Geometry check sheet. Reference: drawing and pictorial views, mm from the part's lowest x, y, z. Round coordinates to 2 decimals unless told otherwise and drop trailing zeros. Write each loop counter-clockwise with the first axis right and the second up, starting at its lowest first coordinate (ties: lowest second). Pieces come first, ordered by that corner, then holes. Notation, with made-up numbers: M 77,38.25 L 128,38.25 A34 cw 128,76.25 Z; hole C -5,85.5 d5. An arc over 180 degrees is marked long. Answer in a Markdown table with one row per item. Add a question column.
1. Material ranges on probe 1 along Z at (x, y) = (38.16, 2.05); probe 2 along X at (y, z) = (0.9, 69); probe 3 along X at (y, z) = (2.55, 71.5), recorded low to high.
2. Go/stop test with flat-tipped pins: pin 1 Ø4 at (x, z) = (50, 31) entering from -Y; pin 2 Ø4.5 at (x, z) = (10.949, 69.94) entering from -Y. Record where each tip stops, or that it passes through.
3. Sectioned sample at B-B on x = 38.16. Record the cut outline in (y, z), plus the area to 3 significant figures.
4. Sectioned sample at A-A on z = 69.94. Record the cut outline in (x, y), plus the area to 3 significant figures.
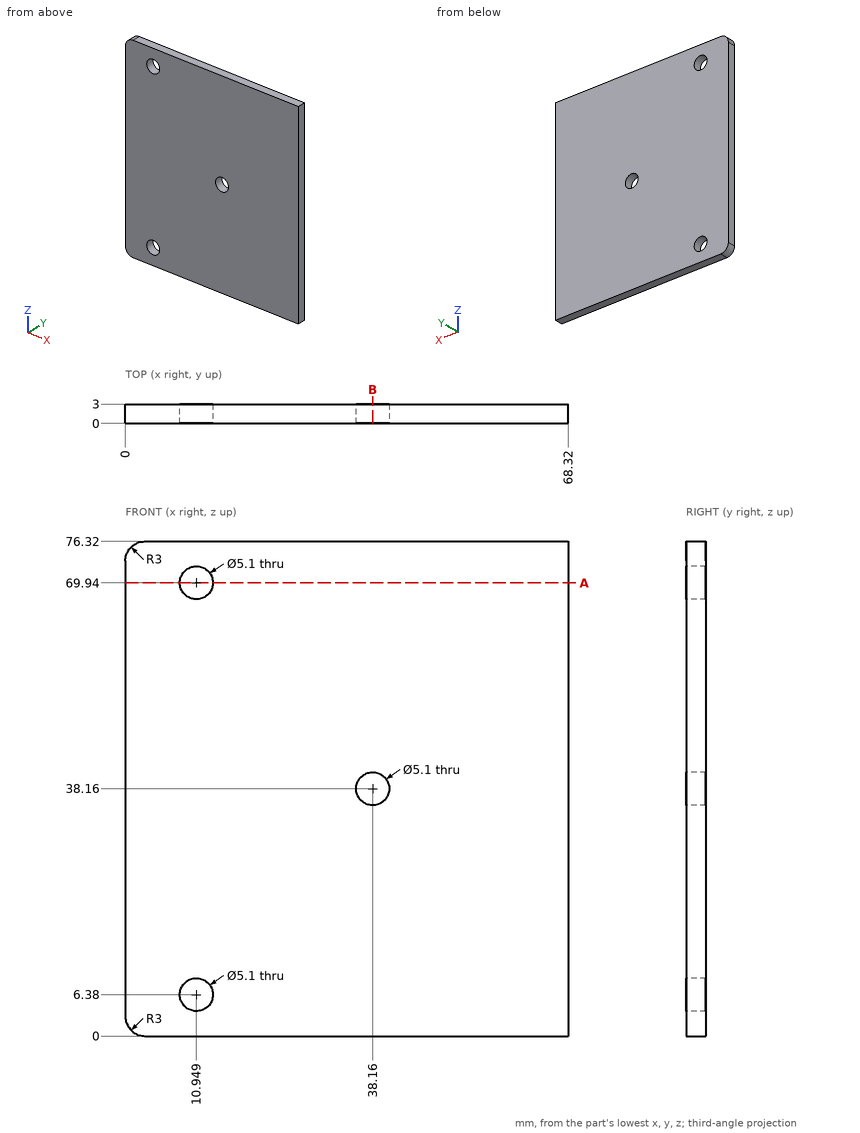
Geometry check:
| question | item | result |
|---|---|---|
| 1 | probe 1 | z = 0 to 35.61, 40.71 to 76.32 |
| 1 | probe 2 | x = 0 to 8.58, 13.32 to 68.32 |
| 1 | probe 3 | x = 0 to 8.93, 12.97 to 68.32 |
| 2 | pin 1 | stops at y = 0 |
| 2 | pin 2 | passes through |
| 3 | outline | M 0,0 L 3,0 L 3,35.61 L 0,35.61 Z; M 0,40.71 L 3,40.71 L 3,76.32 L 0,76.32 Z |
| 3 | area | 214 mm2 |
| 4 | outline | M 0,0 L 8.4,0 L 8.4,3 L 0,3 Z; M 13.5,0 L 68.32,0 L 68.32,3 L 13.5,3 Z |
| 4 | area | 190 mm2 |
